Work out the finished part from the listing and answer in its coordinate system (mm). A direction names the side the tool comes from. Give positions to 0.01 mm unless a question says otherwise; leave off trailing zeros. Order: outer loops, then holes, each group sorted by start corner. A loop starts at its lowest first (then second) coordinate and runs counter-clockwise, first axis right, second up.
```python
from build123d import *

# Parameters (mm, degrees)
SKETCH2_W           = 20
SKETCH2_H           = 50
BOSS_EXTRUDE1_DEPTH = 44.5
SKETCH3_W           = 6.8
SKETCH3_H           = 24.75
SKETCH3_W_2         = 5
SKETCH3_H_2         = 12.5
CUT_EXTRUDE3_DEPTH  = 68.677544282
SKETCH4_R           = 3
SKETCH4_R_2         = 2.6
CUT_EXTRUDE4_DEPTH  = 55.820160525
CUT_EXTRUDE5_REACH  = 56.82
SKETCH4_3_R         = 2.1
BOSS_EXTRUDE2_START = -6.6
SKETCH5_R           = 3
SKETCH5_R_2         = 2.6
BOSS_EXTRUDE2_DEPTH = 6.6
SKETCH6_R           = 3.1
CUT_EXTRUDE6_DEPTH  = 1.23
SKETCH7_W           = 4.6
SKETCH7_H           = 20.1
CUT_EXTRUDE7_DEPTH  = 3.25
FILLET1_R           = 0.5
SKETCH8_R           = 3.35
CUT_EXTRUDE8_DEPTH  = 0.8


with BuildPart() as part:
    # Sketch2 → Boss-Extrude1 (new body)
    with BuildSketch(Plane(origin=(0, 0, 0), x_dir=(1, 0, 0), z_dir=(0, 1, 0))):
        Rectangle(SKETCH2_W, SKETCH2_H)
    extrude(amount=BOSS_EXTRUDE1_DEPTH)

    # Sketch3 → Cut-Extrude3 (cut, through all)
    with BuildSketch(Plane.XY.offset(25)):
        with Locations((0, 32.125)):
            Rectangle(SKETCH3_W, SKETCH3_H)
        with Locations((0, 13.5)):
            Rectangle(SKETCH3_W_2, SKETCH3_H_2)
    extrude(amount=-CUT_EXTRUDE3_DEPTH, mode=Mode.SUBTRACT)

    # Sketch4 → Cut-Extrude4 (cut, through all)
    with BuildSketch(Plane(origin=(10, 0, 0), x_dir=(0, 0, -1), z_dir=(1, 0, 0))):
        with Locations((-13, 32.41)):
            Circle(SKETCH4_R)
        with Locations((12.4, 32.41)):
            Circle(SKETCH4_R_2)
    extrude(amount=-CUT_EXTRUDE4_DEPTH, mode=Mode.SUBTRACT)

    # Sketch4_3 → Cut-Extrude5 (cut, up to next)
    with BuildSketch(Plane(origin=(10, 0, 0), x_dir=(0, 0, -1), z_dir=(1, 0, 0)), mode=Mode.PRIVATE) as cut_extrude5_sk1:
        with Locations((-0.3, 32.41)):
            Circle(SKETCH4_3_R)
    cut_extrude5_tool1 = extrude(cut_extrude5_sk1.sketch, amount=-CUT_EXTRUDE5_REACH, mode=Mode.PRIVATE) & part.part
    # Sketch4_3 → Cut-Extrude5 (cut, up to next)
    with BuildSketch(Plane(origin=(10, 0, 0), x_dir=(0, 0, -1), z_dir=(1, 0, 0)), mode=Mode.PRIVATE) as cut_extrude5_sk2:
        with Locations((-19.35, 38.76)):
            Circle(SKETCH4_3_R)
    cut_extrude5_tool2 = extrude(cut_extrude5_sk2.sketch, amount=-CUT_EXTRUDE5_REACH, mode=Mode.PRIVATE) & part.part
    # Sketch4_3 → Cut-Extrude5 (cut, up to next)
    with BuildSketch(Plane(origin=(10, 0, 0), x_dir=(0, 0, -1), z_dir=(1, 0, 0)), mode=Mode.PRIVATE) as cut_extrude5_sk3:
        with Locations((-6.65, 38.76)):
            Circle(SKETCH4_3_R)
    cut_extrude5_tool3 = extrude(cut_extrude5_sk3.sketch, amount=-CUT_EXTRUDE5_REACH, mode=Mode.PRIVATE) & part.part
    # Sketch4_3 → Cut-Extrude5 (cut, up to next)
    with BuildSketch(Plane(origin=(10, 0, 0), x_dir=(0, 0, -1), z_dir=(1, 0, 0)), mode=Mode.PRIVATE) as cut_extrude5_sk4:
        with Locations((6.05, 38.76)):
            Circle(SKETCH4_3_R)
    cut_extrude5_tool4 = extrude(cut_extrude5_sk4.sketch, amount=-CUT_EXTRUDE5_REACH, mode=Mode.PRIVATE) & part.part
    # Sketch4_3 → Cut-Extrude5 (cut, up to next)
    with BuildSketch(Plane(origin=(10, 0, 0), x_dir=(0, 0, -1), z_dir=(1, 0, 0)), mode=Mode.PRIVATE) as cut_extrude5_sk5:
        with Locations((18.75, 38.76)):
            Circle(SKETCH4_3_R)
    cut_extrude5_tool5 = extrude(cut_extrude5_sk5.sketch, amount=-CUT_EXTRUDE5_REACH, mode=Mode.PRIVATE) & part.part
    # Sketch4_3 → Cut-Extrude5 (cut, up to next)
    with BuildSketch(Plane(origin=(10, 0, 0), x_dir=(0, 0, -1), z_dir=(1, 0, 0)), mode=Mode.PRIVATE) as cut_extrude5_sk6:
        with Locations(Location((18.75, 26.06, 0), (0, 0, 270))):
            Circle(SKETCH4_3_R)
    cut_extrude5_tool6 = extrude(cut_extrude5_sk6.sketch, amount=-CUT_EXTRUDE5_REACH, mode=Mode.PRIVATE) & part.part
    # Sketch4_3 → Cut-Extrude5 (cut, up to next)
    with BuildSketch(Plane(origin=(10, 0, 0), x_dir=(0, 0, -1), z_dir=(1, 0, 0)), mode=Mode.PRIVATE) as cut_extrude5_sk7:
        with Locations(Location((6.05, 26.06, 0), (0, 0, 270))):
            Circle(SKETCH4_3_R)
    cut_extrude5_tool7 = extrude(cut_extrude5_sk7.sketch, amount=-CUT_EXTRUDE5_REACH, mode=Mode.PRIVATE) & part.part
    # Sketch4_3 → Cut-Extrude5 (cut, up to next)
    with BuildSketch(Plane(origin=(10, 0, 0), x_dir=(0, 0, -1), z_dir=(1, 0, 0)), mode=Mode.PRIVATE) as cut_extrude5_sk8:
        with Locations(Location((-6.65, 26.06, 0), (0, 0, 270))):
            Circle(SKETCH4_3_R)
    cut_extrude5_tool8 = extrude(cut_extrude5_sk8.sketch, amount=-CUT_EXTRUDE5_REACH, mode=Mode.PRIVATE) & part.part
    # Sketch4_3 → Cut-Extrude5 (cut, up to next)
    with BuildSketch(Plane(origin=(10, 0, 0), x_dir=(0, 0, -1), z_dir=(1, 0, 0)), mode=Mode.PRIVATE) as cut_extrude5_sk9:
        with Locations(Location((-19.35, 26.06, 0), (0, 0, 270))):
            Circle(SKETCH4_3_R)
    cut_extrude5_tool9 = extrude(cut_extrude5_sk9.sketch, amount=-CUT_EXTRUDE5_REACH, mode=Mode.PRIVATE) & part.part
    add(cut_extrude5_tool1.solids().sort_by_distance((10, 32.41, 0.3))[0], mode=Mode.SUBTRACT)
    add(cut_extrude5_tool2.solids().sort_by_distance((10, 38.76, 19.35))[0], mode=Mode.SUBTRACT)
    add(cut_extrude5_tool3.solids().sort_by_distance((10, 38.76, 6.65))[0], mode=Mode.SUBTRACT)
    add(cut_extrude5_tool4.solids().sort_by_distance((10, 38.76, -6.05))[0], mode=Mode.SUBTRACT)
    add(cut_extrude5_tool5.solids().sort_by_distance((10, 38.76, -18.75))[0], mode=Mode.SUBTRACT)
    add(cut_extrude5_tool6.solids().sort_by_distance((10, 26.06, -18.75))[0], mode=Mode.SUBTRACT)
    add(cut_extrude5_tool7.solids().sort_by_distance((10, 26.06, -6.05))[0], mode=Mode.SUBTRACT)
    add(cut_extrude5_tool8.solids().sort_by_distance((10, 26.06, 6.65))[0], mode=Mode.SUBTRACT)
    add(cut_extrude5_tool9.solids().sort_by_distance((10, 26.06, 19.35))[0], mode=Mode.SUBTRACT)

    # Sketch5 → Boss-Extrude2 (add)
    with BuildSketch(Plane.ZY.offset(10).offset(BOSS_EXTRUDE2_START)):
        with Locations(Location((13, 32.41, 0), (0, 0, 180))):
            Circle(SKETCH5_R)
        with Locations((13, 32.41)):
            Circle(SKETCH5_R_2, mode=Mode.SUBTRACT)
    extrude(amount=BOSS_EXTRUDE2_DEPTH)

    # Sketch6 → Cut-Extrude6 (cut)
    with BuildSketch(Plane.ZY.offset(-3.4)):
        with Locations(Location((-18.75, 26.06, 0), (0, 0, 270))):
            Circle(SKETCH6_R)
        with Locations(Location((-18.75, 38.76, 0), (0, 0, 270))):
            Circle(SKETCH6_R)
        with Locations(Location((-6.05, 38.76, 0), (0, 0, 270))):
            Circle(SKETCH6_R)
        with Locations(Location((6.65, 38.76, 0), (0, 0, 270))):
            Circle(SKETCH6_R)
        with Locations(Location((0.3, 32.41, 0), (0, 0, 270))):
            Circle(SKETCH6_R)
        with Locations(Location((-6.05, 26.06, 0), (0, 0, 270))):
            Circle(SKETCH6_R)
        with Locations(Location((6.65, 26.06, 0), (0, 0, 270))):
            Circle(SKETCH6_R)
        with Locations(Location((19.35, 26.06, 0), (0, 0, 270))):
            Circle(SKETCH6_R)
        with Locations(Location((19.35, 38.76, 0), (0, 0, 270))):
            Circle(SKETCH6_R)
    extrude(amount=-CUT_EXTRUDE6_DEPTH, mode=Mode.SUBTRACT)

    # Sketch7 → Cut-Extrude7 (cut)
    with BuildSketch(Plane.ZY.offset(10)):
        with Locations((-16.3, 13.53)):
            Rectangle(SKETCH7_W, SKETCH7_H)
    extrude(amount=-CUT_EXTRUDE7_DEPTH, mode=Mode.SUBTRACT)

    # Fillet1
    fillet1_edges = [part.edges().sort_by_distance(p)[0] for p in [
        (-10, 44.5, 0),
        (-6.7, 44.5, -25),
        (6.7, 44.5, 25),
        (-6.7, 44.5, 25),
        (0, 7.25, -25),
        (-2.5, 13.5, 25),
        (2.5, 13.5, -25),
        (2.5, 19.75, 0),
        (-2.5, 13.5, -25),
        (3.4, 32.125, -25),
        (0, 7.25, 25),
        (2.5, 13.5, 25),
        (2.95, 19.75, 25),
        (-3.4, 32.125, 25),
        (-2.95, 19.75, 25),
        (-3.4, 44.5, 0),
        (3.4, 32.125, 25),
        (3.4, 44.5, 0),
        (-3.4, 32.125, -25),
        (-2.95, 19.75, -25),
        (-2.5, 19.75, 0),
        (2.95, 19.75, -25),
        (10, 44.5, 0),
        (0, 0, 25),
        (-10, 0, 0),
        (0, 0, -25),
        (10, 0, 0),
        (10, 22.25, 25),
        (-10, 22.25, 25),
        (-10, 22.25, -25),
        (10, 22.25, -25),
        (6.7, 44.5, -25),
    ]]
    fillet(fillet1_edges, radius=FILLET1_R)

    # Sketch8 → Cut-Extrude8 (cut)
    with BuildSketch(Plane(origin=(10, 0, 0), x_dir=(0, 0, -1), z_dir=(1, 0, 0))):
        with Locations((-19.35, 38.76)):
            Circle(SKETCH8_R)
        with Locations((-6.65, 38.76)):
            Circle(SKETCH8_R)
        with Locations((6.05, 38.76)):
            Circle(SKETCH8_R)
        with Locations((18.75, 38.76)):
            Circle(SKETCH8_R)
        with Locations((-0.3, 32.41)):
            Circle(SKETCH8_R)
        with Locations((-19.35, 26.06)):
            Circle(SKETCH8_R)
        with Locations((-6.65, 26.06)):
            Circle(SKETCH8_R)
        with Locations((6.05, 26.06)):
            Circle(SKETCH8_R)
        with Locations((18.75, 26.06)):
            Circle(SKETCH8_R)
    extrude(amount=-CUT_EXTRUDE8_DEPTH, mode=Mode.SUBTRACT)


solid = part.part
```
1. The part is cut by section A-A (x = 8.25). State how many separate pieces and enclosed holes the cut face has, then the cut area to 3 significant figures.
Findings below:
separate pieces: 1
enclosed holes: 11
area: 2,050 mm2
2. The mould has two halves that part along Z. Classify faces 5 (the face through (2.5, 13, 0)), 6 (the face through (9.2, 36.6, -6.7)), 7 (the face through (4.1, 21.9, 25)): pulls with the +Z half, pulls with the -Z half, needs draft (parallel to the pull), parting line crosses it, or undercut.
Findings below:
face 5: needs draft
face 6: undercut
face 7: pulls with the +Z half
3. Which of the six approach directions +Z, -Z, +X, -X, +Y, -Y give full straight-line access (tool end or side, diameter ignored) to faces 1 (the face through (9.2, 28, -20)), 2 (the face through (-2.5, 13, 0)), 3 (the face through (4.006, 29.157, -5.914)), 4 (the face through (-8, 23.58, -16))?
Findings below:
face 1: +X
face 2: +Z, -Z, +Y
face 3: none
face 4: -X
4. Straight lines are drawn through the part: probe 1 along Z at (x, y) = (5.75, 26.06); probe 2 along Z at (x, y) = (4.1, 38.76); probe 3 along Y at (x, z) = (9.6, 6.65). For each, find the intervals that lie inside material, in ascending order.
Findings below:
probe 1: z = -25 to -20.85, -16.65 to -8.15, -3.95 to 4.55, 8.75 to 17.25, 21.45 to 25
probe 2: z = -25 to -21.85, -15.65 to -9.15, -2.95 to 3.55, 9.75 to 16.25, 22.45 to 25
probe 3: y = 0.01 to 22.71, 29.41 to 35.41, 42.11 to 44.49
5. The part is cut by section D-D (x = -8.5). Write down the section's boundary in (y, z), then the cut area to 3 significant figures.
Findings below:
outline: (0, -24.5) arc R0.5 ccw to (0.5, -25) - (44, -25) arc R0.5 ccw to (44.5, -24.5) - (44.5, 24.5) arc R0.5 ccw to (44, 25) - (0.5, 25) arc R0.5 ccw to (0, 24.5) - close; hole (3.48, -18.6) - (23.58, -18.6) - (23.58, -14) - (3.48, -14) - close; hole circle Ø5.2 at (32.41, -12.4); hole circle Ø5.2 at (32.41, 13)
area: 2,090 mm2
6. The part is cut by section B-B (z = -12.4). Write down the section's boundary in (x, y).
Findings below:
outline: (-10, 0.5) arc R0.5 ccw to (-9.5, 0) - (9.5, 0) arc R0.5 ccw to (10, 0.5) - (10, 29.81) - (3.4, 29.81) - (3.4, 19.75) - (3, 19.75) arc R0.5 ccw to (2.5, 19.25) - (2.5, 7.25) - (-2.5, 7.25) - (-2.5, 19.25) arc R0.5 ccw to (-3, 19.75) - (-3.4, 19.75) - (-3.4, 29.81) - (-10, 29.81) - close; (-10, 35.01) - (-3.4, 35.01) - (-3.4, 44) arc R0.5 ccw to (-3.9, 44.5) - (-9.5, 44.5) arc R0.5 ccw to (-10, 44) - close; (3.4, 35.01) - (10, 35.01) - (10, 44) arc R0.5 ccw to (9.5, 44.5) - (3.9, 44.5) arc R0.5 ccw to (3.4, 44) - close
7. Given P1, Ø5, axis at y = 26.06, z = -6.05, coming from the +X side; P2, Ø1.5, axis at x = -3, y = 33, coming from the +Z side; P3, Ø4, axis at y = 38.76, z = -6.05, coming from the +X side, each flat-ended and moving along its own axis, determine where each tip first touches the part or whether it passes through.
Findings below:
P1: stops at x = 9.2
P2: stops at z = 24.98
P3: stops at x = -3.4
8. The part is cut by section C-C (y = 9.5). Write down the section's boundary in (x, z).
Findings below:
outline: (-10, -24.5) arc R0.5 ccw to (-9.5, -25) - (-3, -25) arc R0.5 ccw to (-2.5, -24.5) - (-2.5, 24.5) arc R0.5 ccw to (-3, 25) - (-9.5, 25) arc R0.5 ccw to (-10, 24.5) - (-10, -14) - (-6.75, -14) - (-6.75, -18.6) - (-10, -18.6) - close; (2.5, -24.5) arc R0.5 ccw to (3, -25) - (9.5, -25) arc R0.5 ccw to (10, -24.5) - (10, 24.5) arc R0.5 ccw to (9.5, 25) - (3, 25) arc R0.5 ccw to (2.5, 24.5) - close
